Check sheet for the modelled part. Datum: model origin and axes. Units: mm. Face numbers are marked on the shaded views. A direction names the side the tool comes from. Give positions to 0.01 mm unless a question says otherwise; leave off trailing zeros. Loops run counter-clockwise (first coordinate to the right, second up) from the corner with the lowest first, then second, coordinate; pieces in that order, holes last. Notation, with made-up numbers: (2, 27) -> (48, 27) arc R20 ccw to (48, 52) -> close; hole circle Ø5 at (-6.75, 59.25). An arc over 180 degrees is marked (long way). Write each question's results on one line, items separated by ' | '. Start each with the question number.
1. Tool access check on the marked faces 5 and 6. Record the directions out of +Z, -Z, +X, -X, +Y, -Y that give a thin tool (end or side, any length) a straight path to the whole face; none if there is none.
2. Gauge pin test, flat ends, axial feed: pin 1 Ø5.5 at (x, z) = (35.5, 18.5) entering from +Y; pin 2 Ø1.5 at (x, z) = (-16, 24.5) entering from +Y. Record the tip position at first contact, or that the pin passes through.
3. Cross-section at A-A on x = -24.5. Record the boundary of the cut face in (y, z).
4. Cross-section at D-D on x = 42. Record the boundary of the cut face in (y, z), and give its area (3 significant figures).
5. Mould release check, pull along X, two halves, no side actions. Record for the marked faces 1, 2, 3 and 4: +X half, -X half, draft (parallel to the pull), parting line (faces both ways), or undercut.
6. Cross-section at B-B on y = 12. Record the boundary of the cut face in (x, z).
7. Cross-section at C-C on z = 30. Record the boundary of the cut face in (x, y).
8. Material ranges on L1, parallel to X at y = 16, z = 17; L2, parallel to X at y = 26.5, z = 41; L3, parallel to Y at x = -3, z = 30.5, recorded low to high. Write a range as from..to.
Autodesk Inventor part; units mm, degrees
ref_plane "YZ Plane" through (0, 0, 0) normal (1, 0, 0) x (0, 1, 0)
ref_plane "XZ Plane" through (0, 0, 0) normal (0, 1, 0) x (-1, 0, 0)
ref_plane "XY Plane" through (0, 0, 0) normal (0, 0, 1) x (1, 0, 0)
sketch "Sketch1" plane through (0, 0, 0) normal (0, 0, 1) x (1, 0, 0)
  line L0 (-31.6809, 29.4017) -> (48.3191, 29.4017)
  line L1 (48.3191, 29.4017) -> (48.3191, -30.5983)
  line L2 (48.3191, -30.5983) -> (-31.6809, -30.5983)
  line L3 (-31.6809, -30.5983) -> (-31.6809, 29.4017)
  point P0 (0, 0)
  dimension "d0" = 80
  dimension "d1" = 60
extrude "Extrusion1" add sketch "Sketch1" along normal blind 50
sketch "Sketch2" plane through (0, 0, 50) normal (0, 0, 1) x (1, 0, 0)
  line L0 (-19.9929, 29.4017) -> (-5.9929, 29.4017)
  line L1 (-5.9929, 29.4017) -> (-5.9929, 20.4017)
  line L2 (-5.9929, 20.4017) -> (-0.4929, 20.4017)
  line L3 (-0.4929, 20.4017) -> (-0.4929, 10.4017)
  line L4 (-0.4929, 10.4017) -> (-25.4929, 10.4017)
  line L5 (-25.4929, 10.4017) -> (-25.4929, 20.4017)
  line L6 (-25.4929, 20.4017) -> (-19.9929, 20.4017)
  line L7 (-19.9929, 20.4017) -> (-19.9929, 29.4017)
  line L8 (48.3191, 29.4017) -> (-31.6809, 29.4017)
  point P0 (0, 0)
  point P1 (-12.9929, 29.4017)
  dimension "d4" = 25
  dimension "d5" = 12.5
  dimension "d6" = 7
  dimension "d7" = 14
  dimension "d8" = 9
  dimension "d9" = 10
extrude "Extrusion2" cut sketch "Sketch2" against normal blind 50
sketch "Sketch3" plane through (0, 0, 50) normal (0, 0, 1) x (1, 0, 0)
  line L0 (37.593, 29.4385) -> (44.593, 29.4385)
  line L1 (44.593, 29.4385) -> (44.593, 25.8997)
  line L2 (44.593, 25.8997) -> (46.0072, 24.4855)
  line L3 (46.0072, 24.4855) -> (44.593, 23.0713)
  line L4 (44.593, 23.0713) -> (43.2258, 24.4385)
  line L5 (43.2258, 24.4385) -> (37.593, 24.4385)
  line L6 (37.593, 29.4385) -> (37.593, 24.4385) construction
  line L7 (37.593, 29.4385) -> (30.593, 29.4385)
  line L8 (30.593, 29.4385) -> (30.593, 25.8997)
  line L9 (30.593, 25.8997) -> (29.1788, 24.4855)
  line L10 (29.1788, 24.4855) -> (30.593, 23.0713)
  line L11 (30.593, 23.0713) -> (31.9602, 24.4385)
  line L12 (31.9602, 24.4385) -> (37.593, 24.4385)
  point P0 (0, 0)
  point P1 (31.0916, 30.5867)
  dimension "d23" = 7
  dimension "d24" = 2
  dimension "d26" = 2
  dimension "d27" = 135
  dimension "d28" = 5
extrude "Extrusion3" cut sketch "Sketch3" against normal blind 50
properties part number "PiesaSuportCanale"
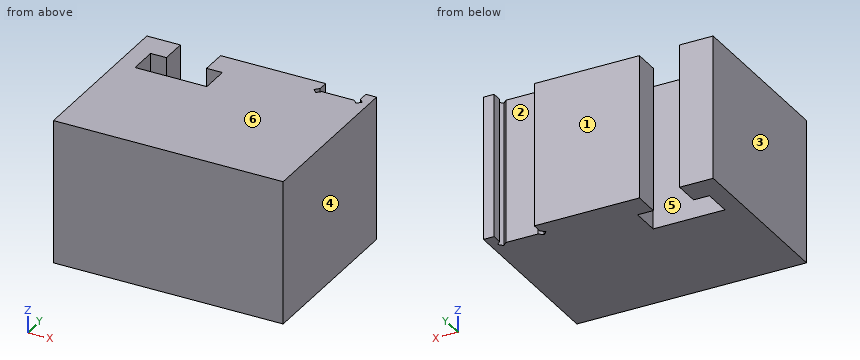
Geometry says:
1) face 5: +Z, -Z | face 6: +Z, +X, -X, +Y, -Y
2) pin 1: y = 24.44 | pin 2: y = 10.4
3) outline: (-30.6, 0) -> (10.4, 0) -> (10.4, 50) -> (-30.6, 50) -> close; (20.4, 0) -> (29.4, 0) -> (29.4, 50) -> (20.4, 50) -> close
4) outline: (-30.6, 0) -> (24.44, 0) -> (24.44, 50) -> (-30.6, 50) -> close | area: 2,750 mm^2
5) face 1: draft | face 2: undercut | face 3: -X half | face 4: +X half
6) outline: (-31.68, 0) -> (-25.49, 0) -> (-25.49, 50) -> (-31.68, 50) -> close; (-0.49, 0) -> (48.32, 0) -> (48.32, 50) -> (-0.49, 50) -> close
7) outline: (-31.68, -30.6) -> (48.32, -30.6) -> (48.32, 29.4) -> (44.59, 29.4) -> (44.59, 25.9) -> (46.01, 24.49) -> (44.59, 23.07) -> (43.23, 24.44) -> (31.96, 24.44) -> (30.59, 23.07) -> (29.18, 24.49) -> (30.59, 25.9) -> (30.59, 29.4) -> (-5.99, 29.4) -> (-5.99, 20.4) -> (-0.49, 20.4) -> (-0.49, 10.4) -> (-25.49, 10.4) -> (-25.49, 20.4) -> (-19.99, 20.4) -> (-19.99, 29.4) -> (-31.68, 29.4) -> close
8) L1: -31.68..-25.49, -0.49..48.32 | L2: -31.68..-19.99, -5.99..30.59, 44.59..48.32 | L3: -30.6..10.4, 20.4..29.4
